Autodesk Inventor part; units mm, degrees
ref_plane "YZ Plane" through (0, 0, 0) normal (1, 0, 0) x (0, 1, 0)
ref_plane "XZ Plane" through (0, 0, 0) normal (0, 1, 0) x (-1, 0, 0)
ref_plane "XY Plane" through (0, 0, 0) normal (0, 0, 1) x (1, 0, 0)
sketch "Sketch2" plane through (0, 0, 0) normal (1, 0, 0) x (0, 1, 0)
  line L0 (0, 0) -> (14, 0)
  line L1 (14, 0) -> (14, -20)
  line L2 (14, -20) -> (0, -20)
  line L3 (0, -20) -> (0, 0)
  circle A0 centre (7, -5) radius 1.75
  circle A1 centre (7, -5) radius 3.5 construction
  point P0 (0, -10)
  point P1 (7, -20)
  dimension "d11" = 20
  dimension "d24" = 14
  dimension "d27" = 3.5
  dimension "d28" = 7
  dimension "d29" = 5
extrude "Extrusion1" add sketch "Sketch2" along normal blind 3
sketch "Sketch3" plane through (3, 0, 0) normal (1, 0, 0) x (0, 0, -1)
  line L0 (0, 0) -> (20, 0)
  line L1 (20, 0) -> (10, 0)
  line L2 (10, 0) -> (10, 5)
  line L3 (10, 5) -> (20, 5)
  line L4 (20, 5) -> (20, 0)
  point P0 (10, 0)
  dimension "d12" = 5
  dimension "d13" = 10
extrude "Extrusion2" add sketch "Sketch3" along normal blind 10
sketch "Sketch4" plane through (3, 5, -10) normal (0, 1, 0) x (1, 0, 0)
  circle A0 centre (5, 5) radius 3
  line L0 (10, 10) -> (10, 0)
  point P0 (-3, -10)
  point P1 (10, 5)
  dimension "d16" = 6
  dimension "d17" = 5
extrude "Extrusion3" cut sketch "Sketch4" against normal through all
properties part number "IRSensorMount"
Here's how the part is built. I have some questions about the finished solid (model axes, mm). A direction names the side the tool comes from. Coordinates: 2 decimals unless noted, no trailing zeros. Write each loop counter-clockwise with the first axis right and the second up, starting at its lowest first coordinate (ties: lowest second). Pieces come first, ordered by that corner, then holes.
1) If we section it at A-A (z = -5): List the corners of the cut face in (x, y) for me.
Filled in:
outline: (0, 0) - (3, 0) - (3, 5.25) - (0, 5.25) - close; (0, 8.75) - (3, 8.75) - (3, 14) - (0, 14) - close
2) Which directions (+Z, -Z, +X, -X, +Y, -Y) give clear straight access to the entire face, cutting with the end or side of a thin tool? Please do faces 1 (the face through (8, 2, -10)), 2 (the face through (9.384, 2.535, -12.338)), 3 (the face through (5.7, 5, -12.7)).
Filled in:
face 1: +Z, +X, +Y, -Y
face 2: +Y, -Y
face 3: +Z, -Z, +X, +Y
3) If I drill on line 1 (Z direction, x = 8, y = 2.7); line 2 (X direction, y = 3.5, z = -15); line 3 (Z direction, x = 0.85, y = 7), over which ranges is the centre line in solid material (lowest first)?
Filled in:
line 1: z = -20 to -18, -12 to -10
line 2: x = 0 to 5, 11 to 13
line 3: z = -20 to -6.75, -3.25 to 0
4) If we section it at B-B (y = 7): List the corners of the cut face in (x, z) for me.
Filled in:
outline: (0, -20) - (3, -20) - (3, -6.75) - (0, -6.75) - close; (0, -3.25) - (3, -3.25) - (3, 0) - (0, 0) - close
5) If we section it at D-D (z = -11.5): List the corners of the cut face in (x, y) for me.
Filled in:
outline: (0, 0) - (13, 0) - (13, 5) - (3, 5) - (3, 14) - (0, 14) - close
6) Thinking about a two-plate mould opening in Z: for faces 4 (the face through (1, 7, 0)), 5 (the face through (0, 7, -10)), 6 (the face through (1.48, 7.81, -3.45)), which applies, +Z half, -Z half, draft (parallel to the pull), parting line (faces both ways), or undercut?
Filled in:
face 4: +Z half
face 5: draft
face 6: undercut
7) If we section it at C-C (y = 4.5): List the corners of the cut face in (x, z) for me.
Filled in:
outline: (0, -20) - (13, -20) - (13, -10) - (3, -10) - (3, 0) - (0, 0) - close; hole circle Ø6 at (8, -15)
8) I'm going to push flat-ended pins straight in: pin 1 (5.5 mm diameter, centred on x = 6.5, y = 2.5, fed in from +Z); pin 2 (3 mm diameter, centred on y = 10.5, z = -15.5, fed in from +X). Where does each tip first touch, or does it pass through?
Filled in:
pin 1: stops at z = -10
pin 2: stops at x = 3
